Input: part model. Units: mm. Frame: model coordinates. A direction names the side the tool comes from. Give positions to 0.01 mm unless a question says otherwise; leave off trailing zeros. Write each loop counter-clockwise with the first axis right and the second up, starting at its lowest first coordinate (ties: lowest second). Pieces come first, ordered by that corner, then holes. Notation, with made-up numbers: (-32.5, 52.5) -> (25.5, 52.5) arc R32 cw to (25.5, 80.5) -> close; hole circle Ø5 at (46, -34.5). An arc over 180 degrees is marked (long way). Answer as a JSON object with one key per item and string values. Group by question number.
from build123d import *

# Parameters (mm, degrees)
SKETCH1_W                = 130
SKETCH1_H                = 97
BOSS_EXTRUDE1_DEPTH      = 70
SKETCH2_W                = 78
SKETCH2_H                = 50
CUT_EXTRUDE1_DEPTH       = 137.1396342
FILLET3_R                = 5
SKETCH3_R                = 5.2
CUT_EXTRUDE2_DEPTH       = 108.131928014
SKETCH4_R                = 6.5
CUT_EXTRUDE3_DEPTH       = 5
FILLET4_R                = 2
F_5_0_5_DIAMETER_HOLE1_D = 6
SKETCH8_W                = 20
SKETCH8_H                = 97
BOSS_EXTRUDE2_DEPTH      = 20
FILLET5_R                = 5
M8_TAPPED_HOLE1_D        = 6.8
F_8_0MM_DOWEL_HOLE1_D    = 8


with BuildPart() as part:
    # Sketch1 → Boss-Extrude1 (new body)
    with BuildSketch(Plane(origin=(0, 0, 0), x_dir=(1, 0, 0), z_dir=(0, 1, 0))):
        Rectangle(SKETCH1_W, SKETCH1_H)
    extrude(amount=BOSS_EXTRUDE1_DEPTH)

    # Sketch2 → Cut-Extrude1 (cut, through all)
    with BuildSketch(Plane.XY.offset(48.5)):
        with Locations((0, 25)):
            Rectangle(SKETCH2_W, SKETCH2_H)
    extrude(amount=-CUT_EXTRUDE1_DEPTH, mode=Mode.SUBTRACT)

    # Fillet3
    fillet3_edges = [part.edges().sort_by_distance(p)[0] for p in [
        (-39, 50, 0),
        (39, 50, 0),
    ]]
    fillet(fillet3_edges, radius=FILLET3_R)

    # Sketch3 → Cut-Extrude2 (cut, through all)
    with BuildSketch(Plane(origin=(0, 70, 0), x_dir=(1, 0, 0), z_dir=(0, 1, 0))):
        with Locations(Location((0, 0, 0), (0, 0, 270))):
            Circle(SKETCH3_R)
    extrude(amount=-CUT_EXTRUDE2_DEPTH, mode=Mode.SUBTRACT)

    # Sketch4 → Cut-Extrude3 (cut)
    with BuildSketch(Plane(origin=(0, 70, 0), x_dir=(1, 0, 0), z_dir=(0, 1, 0))):
        with Locations(Location((0, 0, 0), (0, 0, 270))):
            Circle(SKETCH4_R)
    extrude(amount=-CUT_EXTRUDE3_DEPTH, mode=Mode.SUBTRACT)

    # Fillet4
    fillet4_edges = [part.edges().sort_by_distance(p)[0] for p in [
        (-39, 0, 0),
        (39, 0, 0),
    ]]
    fillet(fillet4_edges, radius=FILLET4_R)

    # Ø5.0 (5) Diameter Hole1 (through all)
    with Locations(Plane(origin=(0, 70, 0), x_dir=(1, 0, 0), z_dir=(0, 1, 0))):
        with Locations((-29, 22.5), (29, 22.5), (29, -22.5), (-29, -22.5)):
            Hole(F_5_0_5_DIAMETER_HOLE1_D / 2)

    # Sketch8 → Boss-Extrude2 (add)
    with BuildSketch(Plane(origin=(0, 70, 0), x_dir=(1, 0, 0), z_dir=(0, 1, 0))):
        with Locations((-75, 0)):
            Rectangle(SKETCH8_W, SKETCH8_H)
    boss_extrude2 = extrude(amount=-BOSS_EXTRUDE2_DEPTH)

    # Mirror1: Boss-Extrude2 across plane
    add(boss_extrude2.mirror(Plane(origin=(0, 0, 0), x_dir=(0, 0, 1), z_dir=(1, 0, 0))))

    # Fillet5
    fillet5_edges = [part.edges().sort_by_distance(p)[0] for p in [
        (65, 50, 0),
        (-65, 50, 0),
    ]]
    fillet(fillet5_edges, radius=FILLET5_R)

    # M8 Tapped Hole1 (through all)
    with Locations(Plane(origin=(0, 70, 0), x_dir=(1, 0, 0), z_dir=(0, 1, 0))):
        with Locations((-75, 38.5), (-75, -38.5), (75, -38.5), (75, 38.5)):
            Hole(M8_TAPPED_HOLE1_D / 2)

    # Ø8.0mm Dowel Hole1 (through all)
    with Locations(Plane(origin=(0, 70, 0), x_dir=(1, 0, 0), z_dir=(0, 1, 0))):
        with Locations((-75, 0), (75, 0)):
            Hole(F_8_0MM_DOWEL_HOLE1_D / 2)


solid = part.part
1. Section B-B (y = 29). Return the cut outline in (x, z), plus the area to 3 significant figures.
2. Section C-C (x = 75). Return the cut outline in (y, z).
3. Mould query, pull axis Z, two halves, no side actions, for faces 6 (the face through (1, 51, 48.5)), 7 (the face through (39, 23, 1)), 8 (the face through (75.44, 59.86, 35.13)). Classes: pulls with the +Z half, pulls with the -Z half, needs draft (parallel to the pull), parting line crosses it, or undercut.
4. Section D-D (y = 61.5). State how many separate pieces and enclosed holes the cut face has, plus the area to 3 significant figures.
5. Section A-A (z = 38.5). Return the cut outline in (x, y).
6. Reachability of faces 1 (the face through (-38, 48, -1)), 2 (the face through (5, 65, 2)), 3 (the face through (65, 22, 1)), 4 (the face through (1.56, 57.6, 4.96)), 5 (the face through (-65, 22, 1)) from +Z, -Z, +X, -X, +Y, -Y: full face, straight path, thin tool, end or side. Return the list, or none.
7. Contact query for flat-ended pins moving along their axis: pin 1 Ø1.5 at (y, z) = (23.5, 7.5) entering from +X; pin 2 Ø8 at (x, y) = (5.5, 45) entering from +Z; pin 3 Ø17 at (x, z) = (0, 0) entering from -Y; pin 4 Ø13.5 at (y, z) = (14.5, 18) entering from -X. Output: stop coordinate, or through.
8. Line query: line 1 (Z direction, x = -75, y = 62); line 2 (X direction, y = 63.5, z = 22.5); line 3 (X direction, y = 65, z = 38.5). Output: solid intervals per line, ascending.
Working result:
{
 "1": {"outline": "(-65, -48.5) -> (-39, -48.5) -> (-39, 48.5) -> (-65, 48.5) -> close; (39, -48.5) -> (65, -48.5) -> (65, 48.5) -> (39, 48.5) -> close", "area": "5,040 mm^2"},
 "2": {"outline": "(50, -48.5) -> (70, -48.5) -> (70, -41.9) -> (50, -41.9) -> close; (50, -35.1) -> (70, -35.1) -> (70, -4) -> (50, -4) -> close; (50, 4) -> (70, 4) -> (70, 35.1) -> (50, 35.1) -> close; (50, 41.9) -> (70, 41.9) -> (70, 48.5) -> (50, 48.5) -> close"},
 "3": {"face 6": "pulls with the +Z half", "face 7": "needs draft", "face 8": "undercut"},
 "4": {"separate pieces": "1", "enclosed holes": "11", "area": "16,000 mm^2"},
 "5": {"outline": "(-85, 50) -> (-78.4, 50) -> (-78.4, 70) -> (-85, 70) -> close; (-71.6, 50) -> (-70, 50) arc R5 cw to (-65, 45) -> (-65, 0) -> (-41, 0) arc R2 ccw to (-39, 2) -> (-39, 45) arc R5 cw to (-34, 50) -> (34, 50) arc R5 cw to (39, 45) -> (39, 2) arc R2 ccw to (41, 0) -> (65, 0) -> (65, 45) arc R5 cw to (70, 50) -> (71.6, 50) -> (71.6, 70) -> (-71.6, 70) -> close; (78.4, 50) -> (85, 50) -> (85, 70) -> (78.4, 70) -> close"},
 "6": {"face 1": "+Z, -Z, -Y", "face 2": "+Y", "face 3": "+Z, -Z, +X, -Y", "face 4": "+Y, -Y", "face 5": "+Z, -Z, -X, -Y"},
 "7": {"pin 1": "stops at x = 65", "pin 2": "passes through", "pin 3": "stops at y = 50", "pin 4": "stops at x = -65"},
 "8": {"line 1": "z = -48.5 to -41.9, -35.1 to -4, 4 to 35.1, 41.9 to 48.5", "line 2": "x = -85 to -32, -26 to 26, 32 to 85", "line 3": "x = -85 to -78.4, -71.6 to 71.6, 78.4 to 85"}
}
